Part model, mm, in its own coordinate system. Face numbers are marked on the shaded views. A direction names the side the tool comes from. Round coordinates to 2 decimals unless told otherwise and drop trailing zeros. Write each loop counter-clockwise with the first axis right and the second up, starting at its lowest first coordinate (ties: lowest second). Pieces come first, ordered by that corner, then holes.
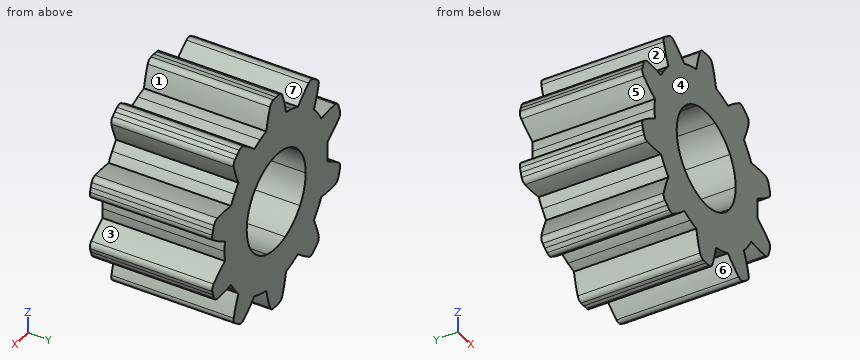
from build123d import *

# Parameters (mm, degrees)
F1_DEPTH = 25
F2_COUNT = 10


with BuildPart() as f1:
    # F0 (on Front) → F1 (new body)
    with BuildSketch(Plane.XZ):
        with BuildLine():
            ThreePointArc((-3.0901699437, 9.510565163), (0, 10), (3.0901699437, 9.510565163))
            Line((3.0901699437, 9.510565163), (5.4077974016, 16.6434890352))
            ThreePointArc((5.4077974016, 16.6434890352), (4.381650071, 16.9425837066), (3.3391574191, 17.1784757103))
            ThreePointArc((3.3391574191, 17.1784757103), (2.8142548796, 19.4430311858), (2.081282357, 21.6490423958))
            ThreePointArc((2.081282357, 21.6490423958), (1.6256906438, 22.2385798355), (0.9212150037, 22.4811334883))
            ThreePointArc((0.9212150037, 22.4811334883), (0.4607040884, 22.4952828776), (0, 22.5))
            ThreePointArc((0, 22.5), (-0.4607040884, 22.4952828776), (-0.9212150037, 22.4811334883))
            ThreePointArc((-0.9212150037, 22.4811334883), (-1.6256906438, 22.2385798355), (-2.081282357, 21.6490423958))
            ThreePointArc((-2.081282357, 21.6490423958), (-2.8142548796, 19.4430311858), (-3.3391574191, 17.1784757103))
            ThreePointArc((-3.3391574191, 17.1784757103), (-4.381650071, 16.9425837066), (-5.4077974016, 16.6434890352))
            Line((-5.4077974016, 16.6434890352), (-3.0901699437, 9.510565163))
        make_face()
    extrude(amount=F1_DEPTH)

    # F2: F1 ×10 about axis
    f2_axis = Axis((0, 0, 0), (0, 1, 0))


with BuildPart() as f1_1:
    add(f1.part)
    for i in range(1, F2_COUNT):
        add(f1.part.rotate(f2_axis, i * 360 / F2_COUNT))


solid = f1_1.part
Q1. Wall check: line 1 (Z direction, x = -0.5, y = -13.25); line 2 (Z direction, x = -19, y = -12.25); line 3 (X direction, y = -23.25, z = 17.5). Give the ranges that are in metal, low to high.
Q2. Two-plate mould, pull along Z, no slides. Class the marked faces 4, 5, 6 and 7: released by +Z, released by -Z, zero draft, split by the parting line, or undercut.
Q3. Tool access for the marked faces 1, 2 and 3: list every direction of +Z, -Z, +X, -X, +Y, -Y with a clear straight run to the whole face (end or side of a thin tool).
Q4. Saw through at C-C, the plane x = 9. Write the cut outline in (y, z).
Q5. Saw through at A-A, the plane x = -6. Write the cut outline in (y, z).
Q6. Drop flat-ended pins along their axis: P1, Ø1, axis at y = -21.5, z = 0.5, coming from the +X side; P2, Ø1.5, axis at x = -2, y = -12, coming from the -Z side; P3, Ø3, axis at x = 13.5, y = -4, coming from the -Z side; P4, Ø6, axis at y = -5, z = 6.5, coming from the -X side. Give the stop position or say it passes through.
Q7. Saw through at B-B, the plane x = 16. Write the cut outline in (y, z).
Computed:
1. line 1: z = -22.49 to -9.99, 9.99 to 22.49
1. line 2: z = -8.7 to -3.1, 3.1 to 8.7
1. line 3: x = -14.12 to -9.3, -3.28 to 3.28, 9.3 to 14.12
2. face 4: zero draft
2. face 5: undercut
2. face 6: released by -Z
2. face 7: released by +Z
3. face 1: +Z, +Y, -Y
3. face 2: -X, +Y, -Y
3. face 3: +X, +Y, -Y
4. outline: (-25, -17.26) - (0, -17.26) - (0, -4.36) - (-25, -4.36) - close; (-25, 4.36) - (0, 4.36) - (0, 17.26) - (-25, 17.26) - close
5. outline: (-25, -16.44) - (0, -16.44) - (0, -8) - (-25, -8) - close; (-25, 8) - (0, 8) - (0, 16.44) - (-25, 16.44) - close
6. P1: stops at x = 17.5
6. P2: stops at z = -22.42
6. P3: stops at z = -18.92
6. P4: stops at x = -21.71
7. outline: (-25, -8.57) - (0, -8.57) - (0, 8.57) - (-25, 8.57) - close
